Geometry: see drawing. Coordinates: mm, zero at the bounding-box minimum. A direction names the side the tool comes from. Coordinates: 2 decimals unless noted, no trailing zeros. Order: outer loops, then holes, each group sorted by start corner. A loop starts at its lowest first (then second) coordinate and runs counter-clockwise, first axis right, second up.
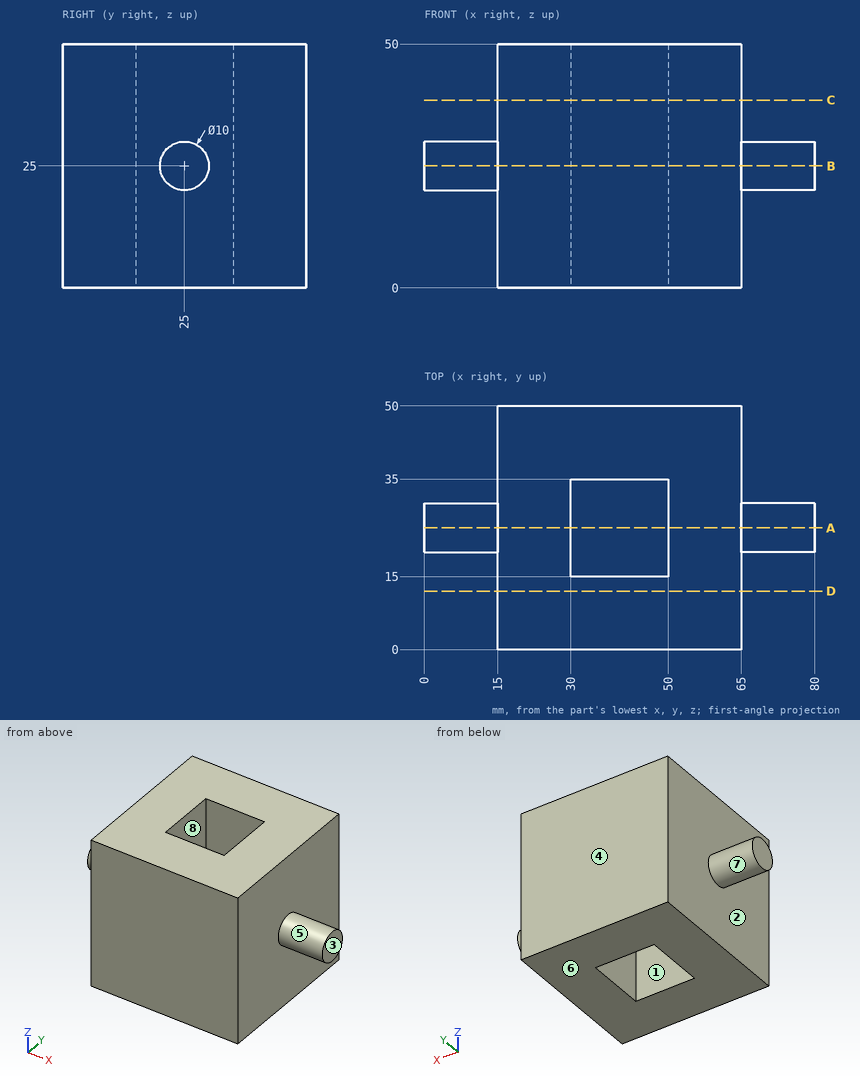
Item 1: Cut plane A-A on y = 25. Return loops of the section in (x, z).
Response values:
outline: (0, 20) - (15, 20) - (15, 0) - (30, 0) - (30, 50) - (15, 50) - (15, 30) - (0, 30) - close; (50, 0) - (65, 0) - (65, 20) - (80, 20) - (80, 30) - (65, 30) - (65, 50) - (50, 50) - close
Item 2: Draft query along X for the marked faces 1, 2 and 3. Return one class per face: pulls with the +X half, pulls with the -X half, needs draft (parallel to the pull), parting line crosses it, or undercut.
Response values:
face 1: undercut
face 2: pulls with the -X half
face 3: pulls with the +X half
Item 3: Access query for the marked faces 4, 5, 6, 7 and 8. Directions: +Z, -Z, +X, -X, +Y, -Y. A direction counts if a zero-diameter tool reaches every point of the face in a straight line with its end or side. Return the directions, or none.
Response values:
face 4: +Z, -Z, +X, -X, +Y
face 5: +X
face 6: -Z, +X, -X, +Y, -Y
face 7: -X
face 8: +Z, -Z
Item 4: Ray query, probe 1 along Y at (x, z) = (39, 30); probe 2 along X at (y, z) = (24, 5.5); probe 3 along X at (y, z) = (9, 14). Return the intervals inside material, ascending.
Response values:
probe 1: y = 0 to 15, 35 to 50
probe 2: x = 15 to 30, 50 to 65
probe 3: x = 15 to 65
Item 5: Cut plane B-B on z = 25. Return loops of the section in (x, y).
Response values:
outline: (0, 20) - (15, 20) - (15, 0) - (65, 0) - (65, 20) - (80, 20) - (80, 30) - (65, 30) - (65, 50) - (15, 50) - (15, 30) - (0, 30) - close; hole (30, 15) - (50, 15) - (50, 35) - (30, 35) - close
Item 6: Pin query (flat end, axial travel): pin 1 Ø6 at (y, z) = (29, 36.5) entering from -X; pin 2 Ø1.5 at (y, z) = (13.5, 40) entering from +X; pin 3 Ø22 at (y, z) = (24, 32) entering from +X. Return the tip coordinate at first contact, or that it passes through.
Response values:
pin 1: stops at x = 15
pin 2: stops at x = 65
pin 3: stops at x = 80
Item 7: Cut plane D-D on y = 12. Return loops of the section in (x, z), then the cut area to 3 significant figures.
Response values:
outline: (15, 0) - (65, 0) - (65, 50) - (15, 50) - close
area: 2,500 mm2
Item 8: Cut plane C-C on z = 38.5. Return loops of the section in (x, y), then the cut area to 3 significant figures.
Response values:
outline: (15, 0) - (65, 0) - (65, 50) - (15, 50) - close; hole (30, 15) - (50, 15) - (50, 35) - (30, 35) - close
area: 2,100 mm2
